Geometry check sheet. Reference: the model listing, model coordinates, mm. A direction names the side the tool comes from. Round coordinates to 2 decimals unless told otherwise and drop trailing zeros. Loops run counter-clockwise (first coordinate to the right, second up) from the corner with the lowest first, then second, coordinate; pieces in that order, holes last.
```python
from build123d import *


with BuildPart() as part:
    # Sketch1 → Revolve1 (revolve)
    with BuildSketch(Plane.XY):
        with BuildLine():
            Line((4, 1.5), (4, -1.5))
            Line((4, -1.5), (8.65, -1.5))
            Line((8.65, -1.5), (10, -1.5))
            Line((10, -1.5), (10, -0.65))
            Line((10, -0.65), (8.65, -0.65))
            ThreePointArc((8.65, -0.65), (8, 0), (8.65, 0.65))
            Line((8.65, 0.65), (10, 0.65))
            Line((10, 0.65), (10, 1.5))
            Line((10, 1.5), (8.65, 1.5))
            Line((8.65, 1.5), (4, 1.5))
        make_face()
    revolve(axis=Axis((0, -1.5, 0), (0, 1, 0)))


solid = part.part
```
1) Sectioned sample at C-C, the plane y = 0.95. Record the cut outline in (x, z).
Report:
outline: circle Ø20 at (0, 0); hole circle Ø8 at (0, 0)
2) Sectioned sample at B-B, the plane z = 0. Record the cut outline in (x, y).
Report:
outline: (-10, -1.5) - (-4, -1.5) - (-4, 1.5) - (-10, 1.5) - (-10, 0.65) - (-8.65, 0.65) arc R0.65 cw to (-8.65, -0.65) - (-10, -0.65) - close; (4, -1.5) - (10, -1.5) - (10, -0.65) - (8.65, -0.65) arc R0.65 cw to (8.65, 0.65) - (10, 0.65) - (10, 1.5) - (4, 1.5) - close
3) Mould release check, pull along Y, two halves, no side actions. Record for faces 3 (the face through (-2.17, -1.07, 9.76)), 4 (the face through (-4.3, -1.5, -0.1)), 5 (the face through (-6, -0.65, -7)): +Y half, -Y half, draft (parallel to the pull), parting line (faces both ways), or undercut.
Report:
face 3: draft
face 4: -Y half
face 5: undercut
4) Sectioned sample at A-A, the plane x = 0. Record the cut outline in (y, z), then the cut area to 3 significant figures.
Report:
outline: (-1.5, -10) - (-0.65, -10) - (-0.65, -8.65) arc R0.65 cw to (0.65, -8.65) - (0.65, -10) - (1.5, -10) - (1.5, -4) - (-1.5, -4) - close; (-1.5, 4) - (1.5, 4) - (1.5, 10) - (0.65, 10) - (0.65, 8.65) arc R0.65 cw to (-0.65, 8.65) - (-0.65, 10) - (-1.5, 10) - close
area: 31.2 mm2
5) Gauge pin test, flat end, axial feed: pin 1 (7 mm diameter, centred on x = 0, z = 0, fed in from -Y). Record the tip position at first contact, or that the pin passes through.
Report:
pin 1: passes through
6) Scan lines: line 1 along Z through (x, y) = (0, -0.75); line 2 along Y through (x, z) = (9, -0.25). Record each from-to range of solid material in increasing order.
Report:
line 1: z = -10 to -4, 4 to 10
line 2: y = -1.5 to -0.65, 0.65 to 1.5
7) Access from +Z, -Z, +X, -X, +Y, -Y to the whole of each face (thin tool, end or side, straight path). Record for faces 1 (the face through (4.3, 1.5, -0.1)), 2 (the face through (6, 0.65, -7)).
Report:
face 1: +Z, -Z, +X, -X, +Y
face 2: none
